Autodesk Inventor part; units mm, degrees
ref_plane "Work Plane1" through (-10, 5, 84) normal (0, 0, 1) x (1, 0, 0)
ref_plane "YZ Plane" through (0, 0, 0) normal (1, 0, 0) x (0, 1, 0)
ref_plane "XZ Plane" through (0, 0, 0) normal (0, 1, 0) x (-1, 0, 0)
sketch "Sketch1" plane through (0, 0, 0) normal (0, 0, 1) x (1, 0, 0)
  line L0 (0, 0) -> (0, 35) construction
  line L1 (0, 35) -> (-10, 35)
  line L2 (-10, 35) -> (-10, 5)
  line L3 (-10, 5) -> (-55, 5)
  line L4 (-55, 5) -> (-55, 35)
  line L5 (-55, 35) -> (-60, 35)
  line L6 (-60, 35) -> (-60, 0)
  line L7 (-60, 0) -> (0, 0)
  line L8 (0, 35) -> (10, 35)
  line L9 (10, 35) -> (10, 5)
  line L10 (10, 5) -> (55, 5)
  line L11 (55, 5) -> (55, 35)
  line L12 (55, 35) -> (60, 35)
  line L13 (60, 35) -> (60, 0)
  line L14 (60, 0) -> (0, 0)
  point P0 (-55, 0)
  point P1 (-10, 0)
  point P2 (55, 0)
  point P3 (10, 0)
  dimension "d0" = 35
  dimension "d1" = 10
  dimension "d2" = 30
  dimension "d3" = 45
  dimension "d4" = 5
extrude "Extrusion1" add sketch "Sketch1" along normal blind 100
sketch "Sketch3" plane through (-60, 0, 0) normal (-1, 0, 0) x (0, 0, 1)
  line L0 (0, 5) -> (100, 5)
  line L1 (0, 35) -> (0, 0)
  line L2 (0, 5) -> (80, 5)
  line L3 (82.5, 5) -> (77.5, 5)
  line L4 (77.5, 5) -> (77.5, 35)
  line L5 (0, 35) -> (100, 35)
  line L6 (82.5, 5) -> (82.5, 35)
  point P0 (82.5, 5)
  point P1 (77.5, 5)
  dimension "d8" = 80
  dimension "d9" = 5
extrude "Extrusion2" cut sketch "Sketch3" against normal through all contours L4 L5 L6 L0
sketch "Sketch4" plane through (-10, 35, 0) normal (0, 1, 0) x (1, 0, 0)
  line L0 (10, 0) -> (10, -50.3)
  line L1 (16.5, -50.3) -> (3.5, -50.3)
  line L2 (3.5, -50.3) -> (3.5, -73.3)
  line L3 (3.5, -73.3) -> (16.5, -73.3)
  line L4 (16.5, -73.3) -> (16.5, -50.3)
  dimension "d12" = 50.3
  dimension "d13" = 13
  dimension "d14" = 23
extrude "Extrusion3" cut sketch "Sketch4" against normal blind 23
sketch "Sketch11" plane through (-10, 35, 77.5) normal (0, 0, 1) x (1, 0, 0)
  line L0 (20, 0) -> (0, 0)
  line L1 (0, 0) -> (10, 0)
  line L2 (10, 0) -> (10, -6.1) construction
  circle A0 centre (10, -6.1) radius 6.3
  line L3 (10, -6.1) -> (10, -12.4) construction
  arc A1 (12.4503, -11.904) -> (10, -9.9) centre (10, -12.4) ccw construction
  arc A2 (7.5497, -11.904) -> (12.4503, -11.904) centre (10, -12.4) ccw
  arc A3 (10, -9.9) -> (7.5497, -11.904) centre (10, -12.4) ccw construction
  line L4 (16.5, 0) -> (16.5, -23)
  line L5 (16.3, -6.1) -> (16.3, 0)
  line L6 (3.7, -6.1) -> (3.7, 0)
  line L7 (3.7, 0) -> (16.3, 0)
  line L8 (16.5, 0) -> (3.5, 0)
  point P0 (10, -35)
  point P1 (3.7, 0)
  dimension "d32" = 10
  dimension "d33" = 6.1
  dimension "d34" = 12.6
  dimension "d35" = 6.3
  dimension "d36" = 5
extrude "Extrusion8" cut sketch "Sketch11" against normal blind 5 contours L5 A0 L0 | A0 L0 | A0 L6 L0 | A2 A0 picked at (7.9397, -7.6935)
sketch "Sketch12" plane through (-60, 0, 0) normal (-1, 0, 0) x (0, 0, 1)
  line L0 (82.5, 35) -> (82.5, 5)
  line L1 (82.5, 35) -> (100, 35)
  line L2 (82.5, 5) -> (90.5, 5)
  line L3 (82.5, 5) -> (100, 5)
  line L4 (90.5, 5) -> (90.5, 35)
  point P0 (0, 0)
  dimension "d39" = 8
extrude "Extrusion9" cut sketch "Sketch12" against normal through all
ref_plane "Work Plane1" through (-10, 5, 84) normal (0, 0, 1) x (1, 0, 0)
sketch "Sketch14" plane through (-10, 35, 0) normal (0, 1, 0) x (1, 0, 0)
  line L0 (5, -45.3) -> (15, -45.3)
  line L1 (15, -45.3) -> (15, -40.3)
  line L2 (15, -40.3) -> (5, -40.3)
  line L3 (5, -40.3) -> (5, -45.3)
  line L4 (0, 0) -> (0, -77.5)
  line L5 (3.5, -50.3) -> (16.5, -50.3)
  point P0 (10, 0)
  point P1 (5, -42.8)
  point P2 (10, -45.3)
  point P3 (10, -50.3)
  dimension "d47" = 10
  dimension "d48" = 5
  dimension "d49" = 5
  dimension "d50" = 5
extrude "Extrusion11" cut sketch "Sketch14" against normal through all
equation "\"d37\" = d36"
properties part number "Selection Body V1_3DPrint"
The model under review builds one solid part; all positions refer to its coordinate system, in mm. A direction names the side the tool comes from. Round coordinates to 2 decimals unless told otherwise and drop trailing zeros. Write each loop counter-clockwise with the first axis right and the second up, starting at its lowest first coordinate (ties: lowest second). Pieces come first, ordered by that corner, then holes. Notation, with made-up numbers: (59, 4) - (82, 4) arc R22 cw to (82, 26) - close; hole circle Ø5 at (43.25, 82.25). An arc over 180 degrees is marked (long way). One line per item, written item: value. Start each with the question number.
1. Consider section A-A on y = 16.5. State how many separate pieces and enclosed holes the cut face has, and give its area (3 significant figures).
2. To check wall thickness, follow L1, parallel to X at y = 7, z = 65.5; L2, parallel to X at y = 22.6, z = 75.25; L3, parallel to X at y = 22, z = 75. State the ranges of each line that lie inside material, in increasing order. Write a range as from..to.
3. Consider section C-C on z = 10. Write out the cut boundary in (x, y).
4. Clearance check with flat-ended pins moving along their axes: P1, Ø8, axis at x = 35, z = 12, coming from the +Y side; P2, Ø10.5, axis at x = 1, z = 57.5, coming from the +Y side. State where each tip first meets the part, or that it passes through.
5. The part is to be moulded in two halves that separate along Z. For faces 1 (the face through (0, 15, 0)), 2 (the face through (-58, 20, 77.5)), 3 (the face through (0, 35, 30)), say which applies: released by +Z, released by -Z, zero draft, split by the parting line, or undercut.
6. Machinability: for faces 4 (the face through (57, 20, 77.5)), 5 (the face through (0, 19, 73.3)), 6 (the face through (0, 18, 40.3)), which of the approach directions +Z, -Z, +X, -X, +Y, -Y give a long, thin tool a straight path to every point of the face, cutting with its end or side? Answer none if there is none.
7. Consider section D-D on z = 58.5. Write out the cut boundary in (x, y).
8. Consider section B-B on x = 0. Write out the cut boundary in (y, z), and give its area (3 significant figures).
Checks:
1. separate pieces: 6
1. enclosed holes: 2
1. area: 2,260 mm^2
2. L1: x = -60..-55, -10..10, 55..60
2. L2: x = -60..-55, -10..-2.5, 2.5..10, 55..60
2. L3: x = -60..-55, -10..-2.43, 2.43..10, 55..60
3. outline: (-60, 0) - (60, 0) - (60, 35) - (55, 35) - (55, 5) - (10, 5) - (10, 35) - (-10, 35) - (-10, 5) - (-55, 5) - (-55, 35) - (-60, 35) - close
4. P1: stops at y = 5
4. P2: stops at y = 12
5. face 1: released by -Z
5. face 2: undercut
5. face 3: zero draft
6. face 4: +X, -X, +Y
6. face 5: +Y
6. face 6: +Y, -Y
7. outline: (-60, 0) - (60, 0) - (60, 35) - (55, 35) - (55, 5) - (10, 5) - (10, 35) - (6.5, 35) - (6.5, 12) - (-6.5, 12) - (-6.5, 35) - (-10, 35) - (-10, 5) - (-55, 5) - (-55, 35) - (-60, 35) - close
8. outline: (0, 0) - (35, 0) - (35, 40.3) - (0, 40.3) - close; (0, 45.3) - (35, 45.3) - (35, 50.3) - (12, 50.3) - (12, 73.3) - (20.1, 73.3) - (20.1, 77.5) - (5, 77.5) - (5, 90.5) - (35, 90.5) - (35, 100) - (0, 100) - close
8. area: 2,340 mm^2
